The listing builds one solid part. Answer for the finished solid, in the listing's coordinates (mm). Face numbers are marked on the shaded views. Coordinates: 2 decimals unless noted, no trailing zeros. Order: outer loops, then holes, each group sorted by start corner. A loop starts at its lowest first (then second) coordinate and runs counter-clockwise, first axis right, second up. Notation, with made-up numbers: (87, 21.25) -> (111, 21.25) arc R15 ccw to (111, 37.25) -> close; hole circle Ø7 at (42, -38). An arc over 180 degrees is marked (long way). Put each result on its own line as item: value. Start each with the question number.
```python
from build123d import *

# Parameters (mm, degrees)
SKETCH1_R           = 2.1
SKETCH1_R_2         = 4.25
BOSS_EXTRUDE1_DEPTH = 5


with BuildPart() as part:
    # Sketch1 → Boss-Extrude1 (new body)
    # profile 1 of 2: a face of its own
    with BuildSketch(Plane.XY):
        with BuildLine():
            Line((-6.331773263, 17), (-30.83030278, 17))
            ThreePointArc((-30.83030278, 17), (-37.5, 0), (-30.83030278, -17))
            Line((-30.83030278, -17), (-6.331773263, -17))
            ThreePointArc((-6.331773263, -17), (5.820650879, -22.382931848), (10, -35))
            ThreePointArc((10, -35), (25, -50), (40, -35))
            ThreePointArc((40, -35), (27.853135577, 0.817900741), (-6.331773263, 17))
        make_face()
        with BuildLine():
            ThreePointArc((34.5, -35), (25, -44.5), (15.5, -35))
            ThreePointArc((15.5, -35), (25, -25.5), (34.5, -35))
        make_face(mode=Mode.SUBTRACT)
        with Locations((-22.5, -13)):
            Circle(SKETCH1_R, mode=Mode.SUBTRACT)
        with Locations((-25, 0)):
            Circle(SKETCH1_R_2, mode=Mode.SUBTRACT)
        with Locations((-2.5, -13)):
            Circle(SKETCH1_R, mode=Mode.SUBTRACT)
        Circle(SKETCH1_R_2, mode=Mode.SUBTRACT)
        with Locations((-22.5, 13)):
            Circle(SKETCH1_R, mode=Mode.SUBTRACT)
        with Locations((-2.5, 13)):
            Circle(SKETCH1_R, mode=Mode.SUBTRACT)
    # profile 2 of 2: a face of its own
    with BuildSketch(Plane.XY):
        with BuildLine():
            ThreePointArc((15.5, -35), (25, -44.5), (34.5, -35))
            ThreePointArc((34.5, -35), (25, -25.5), (15.5, -35))
        make_face()
        with BuildLine():
            ThreePointArc((24.2, -28), (25, -28.8), (25.8, -28))
            ThreePointArc((25.8, -28), (25, -27.2), (24.2, -28))
        make_face(mode=Mode.SUBTRACT)
        with BuildLine():
            ThreePointArc((30.749747468, -30.050252532), (29.949747468, -29.250252532), (29.149747468, -30.050252532))
            ThreePointArc((29.149747468, -30.050252532), (29.949747468, -30.850252532), (30.749747468, -30.050252532))
        make_face(mode=Mode.SUBTRACT)
        with BuildLine():
            ThreePointArc((32.8, -35), (32, -34.2), (31.2, -35))
            ThreePointArc((31.2, -35), (32, -35.8), (32.8, -35))
        make_face(mode=Mode.SUBTRACT)
        with BuildLine():
            ThreePointArc((30.749747468, -39.949747468), (29.949747468, -39.149747468), (29.149747468, -39.949747468))
            ThreePointArc((29.149747468, -39.949747468), (29.949747468, -40.749747468), (30.749747468, -39.949747468))
        make_face(mode=Mode.SUBTRACT)
        with BuildLine():
            ThreePointArc((25.8, -42), (25, -41.2), (24.2, -42))
            ThreePointArc((24.2, -42), (25, -42.8), (25.8, -42))
        make_face(mode=Mode.SUBTRACT)
        with BuildLine():
            ThreePointArc((19.250252532, -39.949747468), (20.050252532, -40.749747468), (20.850252532, -39.949747468))
            ThreePointArc((20.850252532, -39.949747468), (20.050252532, -39.149747468), (19.250252532, -39.949747468))
        make_face(mode=Mode.SUBTRACT)
        with BuildLine():
            ThreePointArc((17.2, -35), (18, -35.8), (18.8, -35))
            ThreePointArc((18.8, -35), (18, -34.2), (17.2, -35))
        make_face(mode=Mode.SUBTRACT)
        with BuildLine():
            ThreePointArc((19.250252532, -30.050252532), (20.050252532, -30.850252532), (20.850252532, -30.050252532))
            ThreePointArc((20.850252532, -30.050252532), (20.050252532, -29.250252532), (19.250252532, -30.050252532))
        make_face(mode=Mode.SUBTRACT)
        with BuildLine():
            ThreePointArc((29.5, -35), (25, -30.5), (20.5, -35))
            ThreePointArc((20.5, -35), (25, -39.5), (29.5, -35))
        make_face(mode=Mode.SUBTRACT)
    extrude(amount=BOSS_EXTRUDE1_DEPTH)


solid = part.part
```
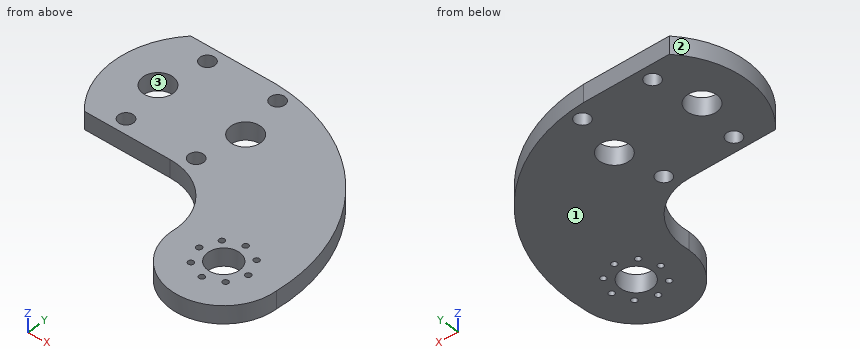
(1) Each of these flat-tipped pins is pushed along its axis until it touches: P1, Ø3, axis at y = -38.5, z = 2.5, coming from the -X side; P2, Ø1.5, axis at x = 26.5, z = 1.5, coming from the +Y side; P3, Ø1.5, axis at x = -21, z = 2.5, coming from the -Y side. Where does it stop, or does it pass through?
(2) For a pull along X with two mould halves and no side action, classify the marked faces 1, 2 and 3 as released by +X, released by -X, zero draft, split by the parting line, or undercut.
(3) The part is cut by section A-A on x = 22.5. Determine the outline of the cut face in (y, z), plus the area to 3 significant figures.
(4) Find the intervals of material crossed by L1, parallel to X at y = 2, z = 4.55; L2, parallel to X at y = -35, z = 3.3; L3, parallel to Y at x = -2.5, z = 2, in increasing order.
(5) The part is cut by section D-D on z = 0.95. Count the separate pieces of the cut face and the enclosed holes in it, plus the area to 3 significant figures.
(6) The part is cut by section B-B on x = -2.5. Determine the outline of the cut face in (y, z).
(7) The part is cut by section C-C on y = 13. Determine the outline of the cut face in (x, z).
Worked out:
1. P1: x = 10.13
1. P2: y = 3.03
1. P3: y = -17
2. face 1: zero draft
2. face 2: released by -X
2. face 3: undercut
3. outline: (-49.79, 0) -> (-38.74, 0) -> (-38.74, 5) -> (-49.79, 5) -> close; (-31.26, 0) -> (5.97, 0) -> (5.97, 5) -> (-31.26, 5) -> close
3. area: 241 mm2
4. L1: -37.42 to -28.75, -21.25 to -3.75, 3.75 to 26.76
4. L2: 10 to 17.2, 18.8 to 20.5, 29.5 to 31.2, 32.8 to 40
4. L3: -17.45 to -15.1, -10.9 to -3.44, 3.44 to 10.9, 15.1 to 16.69
5. separate pieces: 1
5. enclosed holes: 15
5. area: 2,770 mm2
6. outline: (-17.45, 0) -> (-15.1, 0) -> (-15.1, 5) -> (-17.45, 5) -> close; (-10.9, 0) -> (-3.44, 0) -> (-3.44, 5) -> (-10.9, 5) -> close; (3.44, 0) -> (10.9, 0) -> (10.9, 5) -> (3.44, 5) -> close; (15.1, 0) -> (16.69, 0) -> (16.69, 5) -> (15.1, 5) -> close
7. outline: (-33.85, 0) -> (-24.6, 0) -> (-24.6, 5) -> (-33.85, 5) -> close; (-20.4, 0) -> (-4.6, 0) -> (-4.6, 5) -> (-20.4, 5) -> close; (-0.4, 0) -> (11.04, 0) -> (11.04, 5) -> (-0.4, 5) -> close
